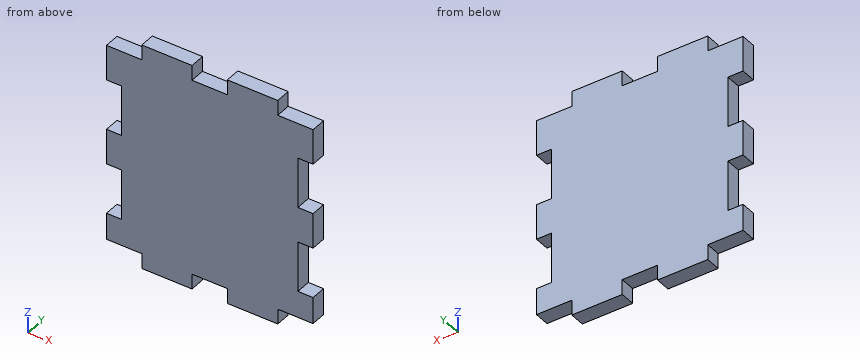
```python
from build123d import *

# Parameters (mm, degrees)
F1_DEPTH = 3


with BuildPart() as f1:
    # F0 (on Front) → F1 (new body)
    with BuildSketch(Plane.XZ):
        Polygon((-7, 1.724721), (0, 1.724721), (0, 7), (-3, 7), (-3, 17), (0, 17), (0, 24), (-3, 24), (-3, 34), (0, 34), (0, 41), (-7, 41), (-7, 44), (-17, 44), (-17, 41), (-24, 41), (-24, 44), (-33.955059, 44), (-33.955059, 41), (-34, 41), (-40.955059, 41), (-40.955059, 34), (-37.955059, 34), (-37.955059, 24), (-40.955059, 24), (-40.955059, 17), (-37.955059, 17), (-37.955059, 7), (-40.955059, 7), (-40.955059, 1.724721), (-34, 1.724721), (-33.955059, 1.724721), (-33.955059, -1.275279), (-24, -1.275279), (-24, 1.724721), (-17, 1.724721), (-17, -1.275279), (-7, -1.275279), align=None)
    extrude(amount=F1_DEPTH)


solid = f1.part
```
Can you work these out from the model? Positions are in its coordinate system, mm. Coordinates: 2 decimals unless noted, no trailing zeros. Order: outer loops, then holes, each group sorted by start corner. A loop starts at its lowest first (then second) coordinate and runs counter-clockwise, first axis right, second up. Notation, with made-up numbers: (72.25, -39.5) - (92.25, -39.5) arc R35 cw to (92.25, -2.5) - close; hole circle Ø2 at (12, -3). An arc over 180 degrees is marked (long way). Answer in a Markdown table with one row per item.
1. If I drill on line 1 along X through (y, z) = (-0.45, 42.5); line 2 along Z through (x, y) = (-39, -1.05); line 3 along X through (y, z) = (-1, 12), over which ranges is the centre line in solid material (lowest first)?
Reply:
| item | result |
|---|---|
| line 1 | x = -33.96 to -24, -17 to -7 |
| line 2 | z = 1.72 to 7, 17 to 24, 34 to 41 |
| line 3 | x = -37.96 to -3 |
2. Suppose I cut it at B-B (z = 12). Please give me the cut outline in (x, y).
Reply:
| item | result |
|---|---|
| outline | (-37.96, -3) - (-3, -3) - (-3, 0) - (-37.96, 0) - close |
3. Suppose I cut it at A-A (x = -21.5). Please give me the cut outline in (y, z).
Reply:
| item | result |
|---|---|
| outline | (-3, 1.72) - (0, 1.72) - (0, 41) - (-3, 41) - close |
4. For pin 1 (1.5 mm diameter, centred on y = -2, z = -0.5, fed in from +X); pin 2 (0.9 mm diameter, centred on x = -19.5, y = -2, fed in from +Z), each with a flat end and sliding along its axis, tell me the tip position at first contact or that it passes through.
Reply:
| item | result |
|---|---|
| pin 1 | stops at x = -7 |
| pin 2 | stops at z = 41 |
